```python
from build123d import *

# Parameters (mm, degrees)
SKETCH1_R           = 2.54
SKETCH1_W           = 50.8
SKETCH1_H           = 355.6
BOSS_EXTRUDE1_DEPTH = 3.175
FILLET1_R           = 6.35
SKETCH6_R           = 2.5
SKETCH6_R_2         = 3.429
SKETCH6_R_3         = 1.905
CUT_EXTRUDE6_DEPTH  = 5.08


with BuildPart() as part:
    # Sketch1 → Boss-Extrude1 (new body)
    # profile 1 of 2: a face of its own
    with BuildSketch(Plane.XY):
        Polygon((0, 190.5), (0, 63.5), (63.5, 63.5), (63.5, 0), (445.262, 0), (445.262, 63.5), (508.762, 63.5), (508.762, 419.1), (280.162, 419.1), align=None)
        with Locations((12.7, 144.4625)):
            Circle(SKETCH1_R, mode=Mode.SUBTRACT)
        with Locations((38.1, 144.4625)):
            Circle(SKETCH1_R, mode=Mode.SUBTRACT)
        with Locations((12.7, 169.8625)):
            Circle(SKETCH1_R, mode=Mode.SUBTRACT)
        with Locations((38.1, 169.8625)):
            Circle(SKETCH1_R, mode=Mode.SUBTRACT)
        with Locations((292.862, 12.7)):
            Circle(SKETCH1_R, mode=Mode.SUBTRACT)
        with Locations((318.262, 12.7)):
            Circle(SKETCH1_R, mode=Mode.SUBTRACT)
        with Locations((292.862, 139.7)):
            Circle(SKETCH1_R, mode=Mode.SUBTRACT)
        with Locations((318.262, 139.7)):
            Circle(SKETCH1_R, mode=Mode.SUBTRACT)
        with Locations((292.862, 266.7)):
            Circle(SKETCH1_R, mode=Mode.SUBTRACT)
        with Locations((318.262, 266.7)):
            Circle(SKETCH1_R, mode=Mode.SUBTRACT)
        with Locations((292.862, 393.7)):
            Circle(SKETCH1_R, mode=Mode.SUBTRACT)
        with Locations((318.262, 393.7)):
            Circle(SKETCH1_R, mode=Mode.SUBTRACT)
    # profile 2 of 2: a face of its own
    with BuildSketch(Plane.XY):
        with Locations((534.162, 241.3)):
            Rectangle(SKETCH1_W, SKETCH1_H)
        with Locations((521.462, 342.9)):
            Circle(SKETCH1_R, mode=Mode.SUBTRACT)
        with Locations((546.862, 342.9)):
            Circle(SKETCH1_R, mode=Mode.SUBTRACT)
        with Locations((521.462, 368.3)):
            Circle(SKETCH1_R, mode=Mode.SUBTRACT)
        with Locations((546.862, 368.3)):
            Circle(SKETCH1_R, mode=Mode.SUBTRACT)
    extrude(amount=BOSS_EXTRUDE1_DEPTH)

    # Fillet1
    fillet1_edges = [part.edges().sort_by_distance(p)[0] for p in [
        (280.162, 419.1, 1.5875),
        (559.562, 419.1, 1.5875),
        (559.562, 63.5, 1.5875),
        (445.262, 63.5, 1.5875),
        (445.262, 0, 1.5875),
        (63.5, 0, 1.5875),
        (63.5, 63.5, 1.5875),
        (0, 63.5, 1.5875),
        (0, 190.5, 1.5875),
    ]]
    fillet(fillet1_edges, radius=FILLET1_R)

    # Sketch6 → Cut-Extrude6 (cut)
    with BuildSketch(Plane(origin=(0, 0, 0), x_dir=(-1, 0, 0), z_dir=(0, 0, -1))):
        with Locations((-507.534100105, 412.722244751)):
            Circle(SKETCH6_R)
        with Locations((-405.934100105, 412.722244751)):
            Circle(SKETCH6_R)
        with Locations((-507.534100105, 196.822244751)):
            Circle(SKETCH6_R)
        with Locations((-513.362102572, 110.957488219)):
            Circle(SKETCH6_R_2)
        with Locations((-456.524599675, 139.527828861)):
            Circle(SKETCH6_R_2)
        with Locations((-405.934100105, 196.822244751)):
            Circle(SKETCH6_R)
        with Locations((-417.19502212, 144.189284242)):
            Circle(SKETCH6_R_3)
        with Locations((-369.44302212, 144.189284242)):
            Circle(SKETCH6_R_3)
        with Locations((-417.192668653, 101.136284242)):
            Circle(SKETCH6_R_3)
        with Locations((-369.44302212, 101.136284242)):
            Circle(SKETCH6_R_3)
    extrude(amount=-CUT_EXTRUDE6_DEPTH, mode=Mode.SUBTRACT)


solid = part.part
```
Here's how the part is built. I have some questions about the finished solid (model axes, mm). Round coordinates to 2 decimals unless told otherwise and drop trailing zeros. Loops run counter-clockwise (first coordinate to the right, second up) from the corner with the lowest first, then second, coordinate; pieces in that order, holes last. Notation, with made-up numbers: (55.25, 9) -> (93.25, 9) arc R23 cw to (93.25, 31) -> close; hole circle Ø10 at (47, -2.75). An arc over 180 degrees is marked (long way). Answer as CSV lines item,"result". Start each with the question number.
1. Imagine slicing it at B-B on x = 259.5. Write out the boundary of the cut face in (y, z) (3 decimals).
2. I'm going to push flat-ended pins straight in: P1, Ø4, axis at x = 507.53, y = 412.72, coming from the +Z side; P2, Ø8, axis at x = 318.262, y = 266.7, coming from the -Z side; P3, Ø1, axis at x = 524.5, z = 1.5, coming from the -Y side. Where does each tip first touch, or does it pass through?
3. Imagine slicing it at A-A on z = 1.8. State how many separate pieces and enclosed holes the cut face has, plus the area to 3 significant figures.
4. I need wall thicknesses on probe 1 along Y at (x, z) = (508, 2.4); probe 2 along X at (y, z) = (342.9, 1.6); probe 3 along X at (y, z) = (368.3, 1.3). Which ranges of each line are inside material? Lowest first, please. Write a range as from..to.
Solution:
1,outline,"(0, 0) -> (402.241, 0) -> (402.241, 3.175) -> (0, 3.175) -> close"
2,P1,"through"
2,P2,"z = 0"
2,P3,"y = 63.5"
3,separate pieces,"1"
3,enclosed holes,"26"
3,area,"191,000 mm²"
4,probe 1,"63.5..194.37, 199.28..410.27, 415.18..419.1"
4,probe 2,"186.77..518.92, 524..544.32, 549.4..559.56"
4,probe 3,"217.9..518.92, 524..544.32, 549.4..559.56"
